Verification items for the finished model (mm, model axes). A direction names the side the tool comes from. Coordinates: 2 decimals unless noted, no trailing zeros. Write each loop counter-clockwise with the first axis right and the second up, starting at its lowest first coordinate (ties: lowest second). Pieces come first, ordered by that corner, then holes. Notation, with made-up numbers: (-20, 9) -> (-12, 9) arc R18 cw to (-12, 32) -> close; hole circle Ø3 at (56, 85.25). An arc over 180 degrees is marked (long way). Write item = value, one per line. Start each with the question number.
(1) Gauge pin test, flat ends, axial feed: pin 1 Ø3 at (x, y) = (-2, -0.5) entering from -Z; pin 2 Ø1.5 at (y, z) = (1.5, 4.5) entering from +X; pin 3 Ø5 at (x, z) = (-4, 6) entering from +Y. Record the tip position at first contact, or that the pin passes through.
(2) Section check D-D (y = -1.5). Record the cut outline in (x, z).
(3) Section check B-B (x = 1.5). Record the cut outline in (y, z).
(4) Material ranges on probe 1 along Z at (x, y) = (4.25, 1.1); probe 2 along X at (y, z) = (-2.2, 7.25); probe 3 along X at (y, z) = (0.7, 6.75), recorded low to high. Write a range as [from, to].
(5) Set-up check for faces 1 (the face through (-10, 0, 5)), 2 (the face through (0.1, 2.5, 10.5)): record each of +Z, -Z, +X, -X, +Y, -Y from which the full face is reachable in a straight line by a thin tool's end or side.
(6) Section check C-C (z = 6). Record the cut outline in (x, y), plus the area to 3 significant figures.
(7) Section check A-A (y = 0). Record the cut outline in (x, z), plus the area to 3 significant figures.
(8) Mould release check, pull along X, two halves, no side actions. Record for faces 3 (the face through (-0.1, -2.5, 10.5)), 4 (the face through (0, 0, 10)): released by +X, released by -X, zero draft, split by the parting line, or undercut.
Autodesk Inventor part; units mm, degrees
ref_plane "YZ Plane" through (0, 0, 0) normal (1, 0, 0) x (0, 1, 0)
ref_plane "XZ Plane" through (0, 0, 0) normal (0, 1, 0) x (-1, 0, 0)
sketch "Sketch1" plane through (0, 0, 0) normal (0, 0, 1) x (1, 0, 0)
  line L0 (-7.5, 2.5) -> (7.5, 2.5)
  line L1 (7.5, -2.5) -> (-7.5, -2.5)
  line L2 (-7.5, 2.5) -> (7.5, -2.5) construction
  line L3 (7.5, 2.5) -> (-7.5, -2.5) construction
  circle A0 centre (-7.5, 0) radius 2.5
  circle A1 centre (7.5, 0) radius 2.5
  point P0 (0, 0)
  point P1 (0, 0)
  point P2 (0, 0)
  dimension "d1" = 5
  dimension "d9" = 7.5
  dimension "d10" = 7.5
extrude "Extrusion1" add sketch "Sketch1" along normal blind 1
extrude "Extrusion2" add sketch "Sketch1" along normal blind 10 contours A0 | A1
ref_plane "Work Plane1" through (0, 0, 11) normal (0, 0, 1) x (1, 0, 0)
sketch "Sketch2" plane through (0, 0, 11) normal (0, 0, 1) x (1, 0, 0)
  arc A0 (7.5, 2.5) -> (7.5, -2.5) centre (7.5, 0) ccw
  line L0 (7.5, 2.5) -> (-7.5, 2.5)
  arc A1 (-7.5, -2.5) -> (-7.5, 2.5) centre (-7.5, 0) ccw
  line L1 (-7.5, -2.5) -> (7.5, -2.5)
  circle A2 centre (-7.5, 0) radius 2.5
  circle A3 centre (7.5, 0) radius 2.5
  point P0 (0, 0)
  point P1 (-7.5, -2.5)
  point P2 (7.5, -2.5)
extrude "Extrusion3" add sketch "Sketch2" against normal blind 1
Response:
q1.pin_1 = 0
q1.pin_2 = 9.88
q1.pin_3 = 2.29
q2.outline = (-9.5, 0) -> (9.5, 0) -> (9.5, 11) -> (-9.5, 11) -> close; hole (-5.5, 1) -> (5.5, 1) -> (5.5, 10) -> (-5.5, 10) -> close
q3.outline = (-2.5, 0) -> (2.5, 0) -> (2.5, 1) -> (-2.5, 1) -> close; (-2.5, 10) -> (2.5, 10) -> (2.5, 11) -> (-2.5, 11) -> close
q4.probe_1 = [0, 1], [10, 11]
q4.probe_2 = [-8.69, -6.31], [6.31, 8.69]
q4.probe_3 = [-9.9, -5.1], [5.1, 9.9]
q5.face_1 = none
q5.face_2 = +Z, -Z, +X, -X, +Y
q6.outline = circle Ø5 at (-7.5, 0); circle Ø5 at (7.5, 0)
q6.area = 39.3 mm2
q7.outline = (-10, 0) -> (10, 0) -> (10, 11) -> (-10, 11) -> close; hole (-5, 1) -> (5, 1) -> (5, 10) -> (-5, 10) -> close
q7.area = 130 mm2
q8.face_3 = zero draft
q8.face_4 = undercut
